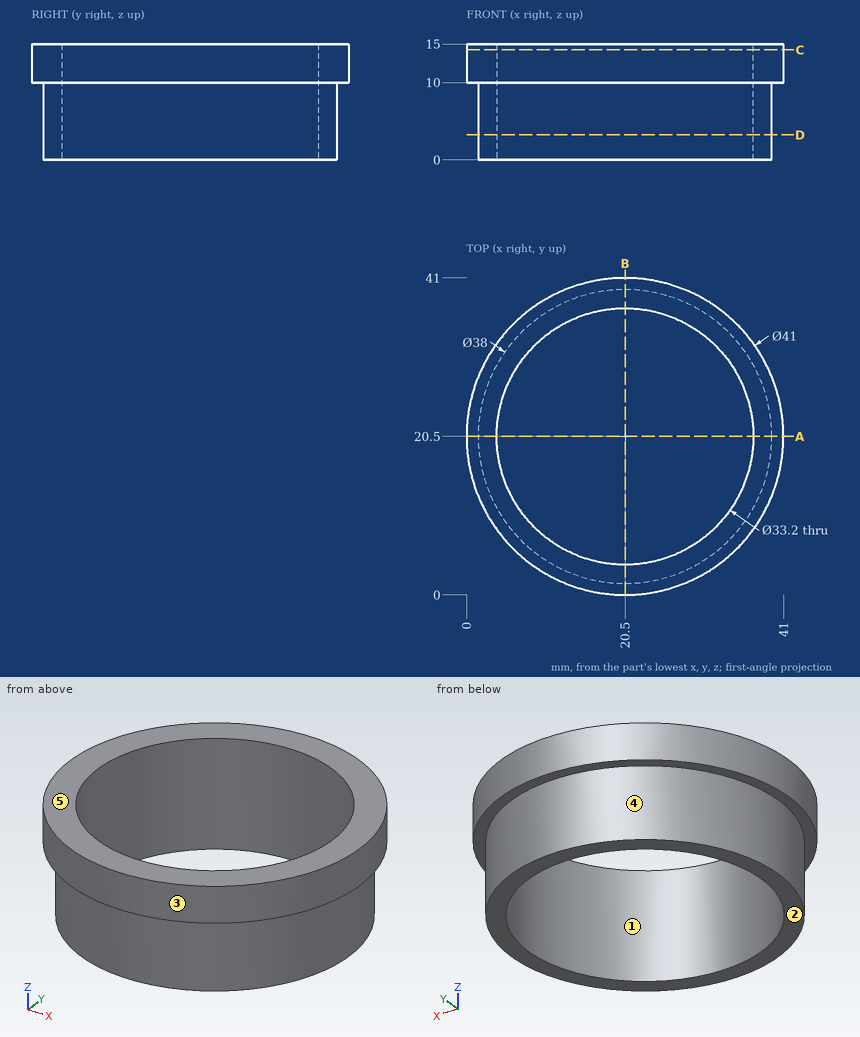
Geometry: see drawing. Coordinates: mm, zero at the bounding-box minimum. A direction names the side the tool comes from. Give positions to 0.01 mm unless a question says otherwise; leave off trailing zeros. Loops run counter-clockwise (first coordinate to the right, second up) from the corner with the lowest first, then second, coordinate; pieces in that order, holes last. Notation, with made-up numbers: (84.5, 18) -> (104.5, 18) arc R15 ccw to (104.5, 22) -> close; hole circle Ø6 at (8.5, 41). An arc over 180 degrees is marked (long way). Use CSV: the item, a comma, the result in double quotes.
(1) Ray query, line 1 along Y through (x, z) = (20.5, 7.25); line 2 along X through (y, z) = (11, 13.25); line 3 along Y through (x, z) = (23, 11). Return the intervals inside material, ascending. Write a range as [from, to].
From the geometry:
line 1,"[1.5, 3.9], [37.1, 39.5]"
line 2,"[2.33, 6.89], [34.11, 38.67]"
line 3,"[0.15, 4.09], [36.91, 40.85]"
(2) Cut plane D-D (z = 3.25). Output: boundary loops of the cut face in (x, y).
From the geometry:
outline,"circle Ø38 at (20.5, 20.5); hole circle Ø33.2 at (20.5, 20.5)"
(3) Access query for the marked faces 4 and 5. Directions: +Z, -Z, +X, -X, +Y, -Y. A direction counts if a zero-diameter tool reaches every point of the face in a straight line with its end or side. Return the directions, or none.
From the geometry:
face 4,"-Z"
face 5,"+Z, +X, -X, +Y, -Y"
(4) First-contact query: P1, Ø4, axis at x = 13, z = 2, coming from the +Y side; P2, Ø8, axis at y = 11, z = 11, coming from the +X side; P3, Ø2, axis at x = 15.5, z = 6.5, coming from the +Y side. Flat tips, straight axial feed; report the tip coordinate or a pass-through.
From the geometry:
P1,"y = 38.69"
P2,"x = 40.25"
P3,"y = 39.07"
(5) Cut plane C-C (z = 14.25). Output: boundary loops of the cut face in (x, y).
From the geometry:
outline,"circle Ø41 at (20.5, 20.5); hole circle Ø33.2 at (20.5, 20.5)"
(6) Cut plane A-A (y = 20.5). Output: boundary loops of the cut face in (x, z).
From the geometry:
outline,"(0, 10) -> (1.5, 10) -> (1.5, 0) -> (3.9, 0) -> (3.9, 15) -> (0, 15) -> close; (37.1, 0) -> (39.5, 0) -> (39.5, 10) -> (41, 10) -> (41, 15) -> (37.1, 15) -> close"
(7) Pull-direction query (X, two-part tool) for the marked faces 1, 2 and 3; classes: released by +X, released by -X, zero draft, split by the parting line, or undercut.
From the geometry:
face 1,"undercut"
face 2,"zero draft"
face 3,"split by the parting line"
